For this review, take the finished solid that the model builds, in its own axes (mm). Give positions to 0.01 mm unless a question says otherwise; leave off trailing zeros. Loops run counter-clockwise (first coordinate to the right, second up) from the corner with the lowest first, then second, coordinate; pieces in that order, holes last. Notation, with made-up numbers: (75.5, -24.5) -> (133.5, -24.5) arc R19 cw to (133.5, 11.5) -> close; hole circle Ø2 at (56, 32). An arc over 180 degrees is marked (long way). One line per question, with ' | ' between items. Start each with the question number.
(1) Wall thickness on probe 1 along Z at (x, y) = (40, 0.5); probe 2 along X at (y, z) = (1, -70); probe 3 along X at (y, z) = (4.15, -46): over which ranges is each line inside the solid? List them lowest first.
(2) Consider section B-B (y = 4.6). Give the number of separate pieces and of enclosed holes in the cut face, and give its area (3 significant figures).
(3) Consider section A-A (z = -46). Write out the cut boundary in (x, y).
from build123d import *

# Parameters (mm, degrees)
SKETCH1_W                  = 86
SKETCH1_H                  = 92
BOSS_EXTRUDE1_DEPTH        = 6
F_7_5_7_5_DIAMETER_HOLE1_D = 7.5
SKETCH6_W                  = 10
SKETCH6_H                  = 6
CUT_EXTRUDE1_DEPTH         = 4
SKETCH61_W                 = 10
SKETCH61_H                 = 6
CUT_EXTRUDE11_DEPTH        = 4
SKETCH62_W                 = 10
SKETCH62_H                 = 6
CUT_EXTRUDE12_DEPTH        = 4
SKETCH64_W                 = 10
SKETCH64_H                 = 6
CUT_EXTRUDE14_DEPTH        = 4
SKETCH65_W                 = 10
SKETCH65_H                 = 6
CUT_EXTRUDE15_DEPTH        = 4
SKETCH66_W                 = 10
SKETCH66_H                 = 6
CUT_EXTRUDE16_DEPTH        = 4
FILLET1_R                  = 5


with BuildPart() as part:
    # Sketch1 → Boss-Extrude1 (new body)
    with BuildSketch(Plane(origin=(0, 0, 0), x_dir=(1, 0, 0), z_dir=(0, 1, 0))):
        with Locations((43, 46)):
            Rectangle(SKETCH1_W, SKETCH1_H)
    extrude(amount=BOSS_EXTRUDE1_DEPTH)

    # Ø7.5 (7.5) Diameter Hole1 (through all)
    with Locations(Plane(origin=(0, 6, 0), x_dir=(1, 0, 0), z_dir=(0, 1, 0))):
        with Locations((71, 46)):
            Hole(F_7_5_7_5_DIAMETER_HOLE1_D / 2)

    # Sketch6 → Cut-Extrude1 (cut, symmetric)
    with BuildSketch(Plane(origin=(9.232221392, 3, 35), x_dir=(1, 0, 0), z_dir=(0, -1, 0))):
        with Locations((0.767778608, -44)):
            Rectangle(SKETCH6_W, SKETCH6_H)
    cut_extrude1 = extrude(amount=CUT_EXTRUDE1_DEPTH, both=True, mode=Mode.SUBTRACT)

    # Sketch61 → Cut-Extrude11 (cut, symmetric)
    with BuildSketch(Plane(origin=(42.232221392, 3, 35), x_dir=(1, 0, 0), z_dir=(0, -1, 0))):
        with Locations((0.767778608, -44)):
            Rectangle(SKETCH61_W, SKETCH61_H)
    cut_extrude11 = extrude(amount=CUT_EXTRUDE11_DEPTH, both=True, mode=Mode.SUBTRACT)

    # Sketch62 → Cut-Extrude12 (cut, symmetric)
    with BuildSketch(Plane(origin=(75.232221392, 3, 35), x_dir=(1, 0, 0), z_dir=(0, -1, 0))):
        with Locations((0.767778608, -44)):
            Rectangle(SKETCH62_W, SKETCH62_H)
    cut_extrude12 = extrude(amount=CUT_EXTRUDE12_DEPTH, both=True, mode=Mode.SUBTRACT)

    # Sketch64 → Cut-Extrude14 (cut, symmetric)
    with BuildSketch(Plane(origin=(9.232221392, 3, 21), x_dir=(1, 0, 0), z_dir=(0, -1, 0))):
        with Locations((0.767778608, -44)):
            Rectangle(SKETCH64_W, SKETCH64_H)
    cut_extrude14 = extrude(amount=CUT_EXTRUDE14_DEPTH, both=True, mode=Mode.SUBTRACT)

    # Sketch65 → Cut-Extrude15 (cut, symmetric)
    with BuildSketch(Plane(origin=(42.232221392, 3, 21), x_dir=(1, 0, 0), z_dir=(0, -1, 0))):
        with Locations((0.767778608, -44)):
            Rectangle(SKETCH65_W, SKETCH65_H)
    cut_extrude15 = extrude(amount=CUT_EXTRUDE15_DEPTH, both=True, mode=Mode.SUBTRACT)

    # Sketch66 → Cut-Extrude16 (cut, symmetric)
    with BuildSketch(Plane(origin=(75.232221392, 3, 21), x_dir=(1, 0, 0), z_dir=(0, -1, 0))):
        with Locations((0.767778608, -44)):
            Rectangle(SKETCH66_W, SKETCH66_H)
    cut_extrude16 = extrude(amount=CUT_EXTRUDE16_DEPTH, both=True, mode=Mode.SUBTRACT)

    # Mirror1: Cut-Extrude1, Cut-Extrude11, Cut-Extrude12, Cut-Extrude14, Cut-Extrude15, Cut-Extrude16 across plane
    add(cut_extrude1.mirror(Plane.XY.offset(-46)), mode=Mode.SUBTRACT)
    add(cut_extrude11.mirror(Plane.XY.offset(-46)), mode=Mode.SUBTRACT)
    add(cut_extrude12.mirror(Plane.XY.offset(-46)), mode=Mode.SUBTRACT)
    add(cut_extrude14.mirror(Plane.XY.offset(-46)), mode=Mode.SUBTRACT)
    add(cut_extrude15.mirror(Plane.XY.offset(-46)), mode=Mode.SUBTRACT)
    add(cut_extrude16.mirror(Plane.XY.offset(-46)), mode=Mode.SUBTRACT)

    # Fillet1
    fillet1_edges = [part.edges().sort_by_distance(p)[0] for p in [
        (0, 3, -92),
        (86, 3, -92),
        (86, 3, 0),
        (0, 3, 0),
    ]]
    fillet(fillet1_edges, radius=FILLET1_R)


solid = part.part
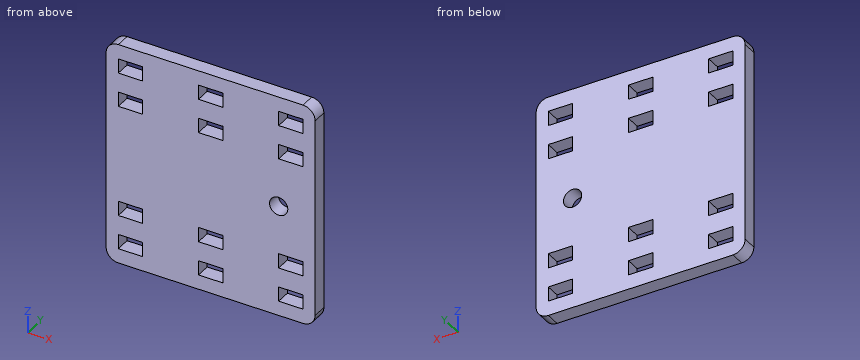
A:
1) probe 1: z = -92 to -86, -80 to -72, -66 to -26, -20 to -12, -6 to 0 | probe 2: x = 0 to 5, 15 to 38, 48 to 71, 81 to 86 | probe 3: x = 0 to 67.25, 74.75 to 86
2) separate pieces: 1 | enclosed holes: 13 | area: 7,130 mm^2
3) outline: (0, 0) -> (67.25, 0) -> (67.25, 6) -> (0, 6) -> close; (74.75, 0) -> (86, 0) -> (86, 6) -> (74.75, 6) -> close
